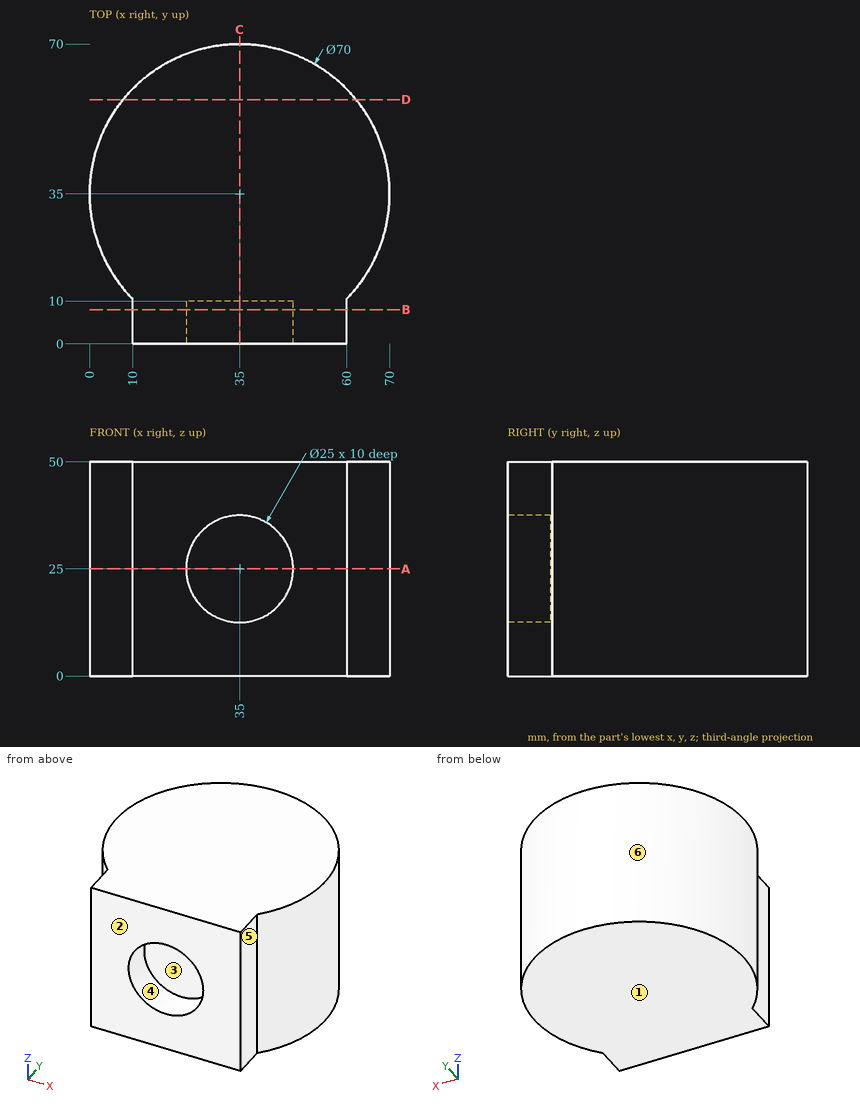
Source: three-view drawing plus pictorial views. Frame: mm from the lowest corner of the part. A direction names the side the tool comes from. Coordinates: 2 decimals unless noted, no trailing zeros. Write each loop counter-clockwise with the first axis right and the second up, starting at its lowest first coordinate (ties: lowest second). Pieces come first, ordered by that corner, then holes. Notation, with made-up numbers: (68, -38.5) - (101, -38.5) arc R17 ccw to (101, -11.5) - close; hole circle Ø3 at (76, 43.5). An arc over 180 degrees is marked (long way). Answer as a JSON object with one key per item and string values.
Q1. Section query C-C, the plane x = 35. Output: boundary loops of the cut face in (y, z).
Ans:
{"outline": "(0, 0) - (70, 0) - (70, 50) - (0, 50) - (0, 37.5) - (10, 37.5) - (10, 12.5) - (0, 12.5) - close"}
Q2. Section query A-A, the plane z = 25. Output: boundary loops of the cut face in (x, y).
Ans:
{"outline": "(10, 0) - (22.5, 0) - (22.5, 10) - (47.5, 10) - (47.5, 0) - (60, 0) - (60, 10.51) arc R35 ccw (long way) to (10, 10.51) - close"}
Q3. First-contact query: pin 1 Ø4 at (x, z) = (38.5, 33) entering from +Y; pin 2 Ø15 at (x, z) = (35, 25) entering from -Y; pin 3 Ø4 at (x, z) = (28, 35.5) entering from +Y. Flat tips, straight axial feed; report the tip coordinate or a pass-through.
Ans:
{"pin 1": "stops at y = 69.97", "pin 2": "stops at y = 10", "pin 3": "stops at y = 69.64"}
Q4. Section query B-B, the plane y = 8. Output: boundary loops of the cut face in (x, z).
Ans:
{"outline": "(10, 0) - (60, 0) - (60, 50) - (10, 50) - close; hole circle Ø25 at (35, 25)"}
Q5. Draft query along Z for the marked faces 1, 2, 3 and 4. Return one class per face: released by +Z, released by -Z, zero draft, split by the parting line, or undercut.
Ans:
{"face 1": "released by -Z", "face 2": "zero draft", "face 3": "undercut", "face 4": "undercut"}
Q6. Section query D-D, the plane y = 57. Output: boundary loops of the cut face in (x, z), plus the area to 3 significant figures.
Ans:
{"outline": "(7.78, 0) - (62.22, 0) - (62.22, 50) - (7.78, 50) - close", "area": "2,720 mm2"}
Q7. Material intervals for line 1 (Z direction, x = 35, y = 5); line 2 (Z direction, x = 44, y = 6.5); line 3 (X direction, y = 35.5, z = 20.5), sorted ascending. Write a range as [from, to].
Ans:
{"line 1": "z = [0, 12.5], [37.5, 50]", "line 2": "z = [0, 16.33], [33.67, 50]", "line 3": "x = [0, 70]"}
Q8. Set-up query: the marked faces 5 and 6. Return all of +Z, -Z, +X, -X, +Y, -Y with unobstructed straight access to the full face (end or side cutting, diameter ignored); none if empty.
Ans:
{"face 5": "+Z, -Z, +X, -Y", "face 6": "+Z, -Z"}
